Could you check a few things on this model? Use its own coordinates, in mm. A direction names the side the tool comes from. Round coordinates to 2 decimals unless told otherwise and drop trailing zeros. Loops run counter-clockwise (first coordinate to the right, second up) from the corner with the lowest first, then second, coordinate; pieces in that order, holes last. Notation, with made-up numbers: M 32,-13.75 L 53,-13.75 A27 ccw 53,19.25 Z; hole C 65,-4.75 d1. An arc over 180 degrees is marked long. Answer in a Markdown table with one row per item.
```python
from build123d import *

# Parameters (mm, degrees)
SKETCH1_W           = 135
SKETCH1_H           = 135
BOSS_EXTRUDE1_DEPTH = 18
FILLET1_R           = 5
SKETCH2_R           = 13
CUT_EXTRUDE1_DEPTH  = 10
CHAMFER1_SIZE       = 2


with BuildPart() as part:
    # Sketch1 → Boss-Extrude1 (new body)
    with BuildSketch(Plane(origin=(0, 0, 0), x_dir=(1, 0, 0), z_dir=(0, 1, 0))):
        Rectangle(SKETCH1_W, SKETCH1_H)
    extrude(amount=BOSS_EXTRUDE1_DEPTH)

    # Fillet1
    fillet1_edges = [part.edges().sort_by_distance(p)[0] for p in [
        (67.5, 9, 67.5),
        (-67.5, 9, 67.5),
        (-67.5, 9, -67.5),
        (67.5, 9, -67.5),
    ]]
    fillet(fillet1_edges, radius=FILLET1_R)

    # Sketch2 → Cut-Extrude1 (cut)
    with BuildSketch(Plane(origin=(0, 18, 0), x_dir=(1, 0, 0), z_dir=(0, 1, 0))):
        with Locations((-49.5, 49.5)):
            Circle(SKETCH2_R)
        with Locations((49.5, 49.5)):
            Circle(SKETCH2_R)
        with Locations((49.5, -49.5)):
            Circle(SKETCH2_R)
        with Locations((-49.5, -49.5)):
            Circle(SKETCH2_R)
        with Locations((-16.5, 49.5)):
            Circle(SKETCH2_R)
        with Locations((16.5, 49.5)):
            Circle(SKETCH2_R)
        with Locations((-16.5, 16.5)):
            Circle(SKETCH2_R)
        with Locations((-49.5, 16.5)):
            Circle(SKETCH2_R)
        with Locations((-16.5, -49.5)):
            Circle(SKETCH2_R)
        with Locations((-49.5, -16.5)):
            Circle(SKETCH2_R)
        with Locations((-16.5, -16.5)):
            Circle(SKETCH2_R)
        with Locations((49.5, 16.5)):
            Circle(SKETCH2_R)
        with Locations((16.5, 16.5)):
            Circle(SKETCH2_R)
        with Locations((49.5, -16.5)):
            Circle(SKETCH2_R)
        with Locations((16.5, -16.5)):
            Circle(SKETCH2_R)
        with Locations((16.5, -49.5)):
            Circle(SKETCH2_R)
    extrude(amount=-CUT_EXTRUDE1_DEPTH, mode=Mode.SUBTRACT)

    # Chamfer1
    chamfer1_edges = [part.edges().sort_by_distance(p)[0] for p in [
        (3.5, 18, -49.5),
        (-29.5, 18, -16.5),
        (-62.5, 18, -16.5),
        (-29.5, 18, 49.5),
        (-29.5, 18, -49.5),
        (-62.5, 18, 49.5),
        (36.5, 18, 49.5),
        (36.5, 18, -49.5),
        (3.5, 18, 49.5),
        (3.5, 18, 16.5),
        (36.5, 18, 16.5),
        (3.5, 18, -16.5),
        (36.5, 18, -16.5),
        (-29.5, 18, 16.5),
        (-62.5, 18, 16.5),
        (-62.5, 18, -49.5),
    ]]
    chamfer(chamfer1_edges, length=CHAMFER1_SIZE)


solid = part.part
```
1) I need wall thicknesses on line 1 (X direction, y = 10.5, z = 16.5); line 2 (Z direction, x = -8.5, y = 15). Which ranges of each line are inside material? Lowest first, please.
Computed:
| item | result |
|---|---|
| line 1 | x = -67.5 to -62.5, -36.5 to -29.5, -3.5 to 3.5, 29.5 to 36.5, 62.5 to 67.5 |
| line 2 | z = -67.5 to -59.75, -39.25 to -26.75, -6.25 to 6.25, 26.75 to 39.25, 59.75 to 67.5 |
2) If we mould it in two halves opening along X, with no side actions, what happens to faces 3 (the face through (-17, 8, 16)), 4 (the face through (-66.07, 9.13, 66)), 5 (the face through (67.5, 9, 1))? For each: released by +X, released by -X, zero draft, split by the parting line, or undercut.
Computed:
| item | result |
|---|---|
| face 3 | undercut |
| face 4 | released by -X |
| face 5 | released by +X |
3) Which directions (+Z, -Z, +X, -X, +Y, -Y) give clear straight access to the entire face, cutting with the end or side of a thin tool? Please do faces 1 (the face through (-17, 8, -17)), 2 (the face through (-1, 18, -1)).
Computed:
| item | result |
|---|---|
| face 1 | +Y |
| face 2 | +Z, -Z, +X, -X, +Y |
4) Will these pins go through, and if not, where does the flat tip stop? P1, Ø8, axis at x = -50.5, z = -45, coming from the +Y side; P2, Ø21, axis at x = -16, z = -52.5, coming from the +Y side.
Computed:
| item | result |
|---|---|
| P1 | stops at y = 8 |
| P2 | stops at y = 16.54 |
5) I want a section at C-C, the plane z = -49.5. Please give me the cut outline in (x, y).
Computed:
| item | result |
|---|---|
| outline | M -67.5,0 L 67.5,0 L 67.5,18 L 64.5,18 L 62.5,16 L 62.5,8 L 36.5,8 L 36.5,16 L 34.5,18 L 31.5,18 L 29.5,16 L 29.5,8 L 3.5,8 L 3.5,16 L 1.5,18 L -1.5,18 L -3.5,16 L -3.5,8 L -29.5,8 L -29.5,16 L -31.5,18 L -34.5,18 L -36.5,16 L -36.5,8 L -62.5,8 L -62.5,16 L -64.5,18 L -67.5,18 Z |
6) I want a section at B-B, the plane y = 12. State how many separate pieces and enclosed holes the cut face has, plus the area to 3 significant figures.
Computed:
| item | result |
|---|---|
| separate pieces | 1 |
| enclosed holes | 16 |
| area | 9,710 mm² |
7) I want a section at A-A, the plane x = 49.5. Please give me the cut outline in (y, z).
Computed:
| item | result |
|---|---|
| outline | M 0,-67.5 L 18,-67.5 L 18,-64.5 L 16,-62.5 L 8,-62.5 L 8,-36.5 L 16,-36.5 L 18,-34.5 L 18,-31.5 L 16,-29.5 L 8,-29.5 L 8,-3.5 L 16,-3.5 L 18,-1.5 L 18,1.5 L 16,3.5 L 8,3.5 L 8,29.5 L 16,29.5 L 18,31.5 L 18,34.5 L 16,36.5 L 8,36.5 L 8,62.5 L 16,62.5 L 18,64.5 L 18,67.5 L 0,67.5 Z |
